Geometry: final body of the model. Coordinates: model frame, mm. A direction names the side the tool comes from. Round coordinates to 2 decimals unless told otherwise and drop trailing zeros. Loops run counter-clockwise (first coordinate to the right, second up) from the corner with the lowest first, then second, coordinate; pieces in that order, holes last. Notation, with made-up numbers: M 4,65 L 62,65 A28 cw 62,93 Z; hole C -1,49 d5. An arc over 180 degrees is marked long. Return JSON: item names as keys, results as strings.
from build123d import *

# Parameters (mm, degrees)
F4_W     = 64.961583
F4_H     = 61.849
F4_W_2   = 38.670417
F4_H_2   = 56.769
F5_DEPTH = 1.524
F1_R     = 3.7973
F1_R_2   = 2.07645
F1_R_3   = 2.286
F6_DEPTH = 4.064
F7_DEPTH = 25.4


with BuildPart() as f5:
    # F4 (on Top) → F5 (new body)
    with BuildSketch(Plane.XY):
        with Locations((-58.240771, 19.304)):
            Rectangle(F4_W, F4_H)
        with Locations((-58.240772, 19.304)):
            Rectangle(F4_W_2, F4_H_2, mode=Mode.SUBTRACT)
    extrude(amount=F5_DEPTH)

    # F1 (on Top) → F6 (join)
    with BuildSketch(Plane.XY):
        with Locations((-84.910771, -5.08)):
            Circle(F1_R)
        with Locations((-84.910771, -5.08)):
            Circle(F1_R_2, mode=Mode.SUBTRACT)
        with Locations((-83.640771, 43.688)):
            Circle(F1_R_3)
        with Locations((-32.840771, 0)):
            Circle(F1_R_3)
        with Locations((-32.840771, 28.448)):
            Circle(F1_R)
        with Locations((-32.840771, 28.448)):
            Circle(F1_R_2, mode=Mode.SUBTRACT)
    extrude(amount=F6_DEPTH)

    # F1 (on Top) → F7 (cut)
    with BuildSketch(Plane.XY):
        with Locations((-84.910771, -5.08)):
            Circle(F1_R_2)
        with Locations((-32.840771, 28.448)):
            Circle(F1_R_2)
    extrude(amount=F7_DEPTH, mode=Mode.SUBTRACT)


solid = f5.part
Q1. Section query D-D (z = 3.25). Output: boundary loops of the cut face in (x, y).
Determined:
{"outline": "C -84.91,-5.08 d7.59; C -83.64,43.69 d4.57; C -32.84,28.45 d7.59; C -32.84,0 d4.57; hole C -84.91,-5.08 d4.15; hole C -32.84,28.45 d4.15"}
Q2. Pin query (flat end, axial travel): pin 1 (10 mm diameter, centred on x = -32.5, y = 13.5, fed in from +Z); pin 2 (2 mm diameter, centred on y = 28.5, z = 3, fed in from -X); pin 3 (1.5 mm diameter, centred on y = 19.5, z = 3, fed in from +X). Return the tip coordinate at first contact, or that it passes through.
Determined:
{"pin 1": "stops at z = 1.52", "pin 2": "stops at x = -36.64", "pin 3": "passes through"}
Q3. Material intervals for L1, parallel to Y at x = -55.5, z = 1.15; L2, parallel to X at y = 8.5, z = 0.65; L3, parallel to Y at x = -83, z = 2.1, sorted ascending.
Determined:
{"L1": "y = -11.62 to -9.08, 47.69 to 50.23", "L2": "x = -90.72 to -77.58, -38.91 to -25.76", "L3": "y = -8.36 to -5.89, -4.27 to -1.8, 41.49 to 45.88"}
Q4. Pull-direction query (Y, two-part tool) for faces 1 (the flat face through (-38.906, 19, 1)), 2 (the flat face through (-59, -11.62, 1)), 3 (the flat face through (-31, 27, 4.064)); classes: pulls with the +Y half, pulls with the -Y half, needs draft (parallel to the pull), parting line crosses it, or undercut.
Determined:
{"face 1": "undercut", "face 2": "pulls with the -Y half", "face 3": "needs draft"}
Q5. Section query B-B (x = -50). Output: boundary loops of the cut face in (y, z), plus the area to 3 significant figures.
Determined:
{"outline": "M -11.62,0 L -9.08,0 L -9.08,1.52 L -11.62,1.52 Z; M 47.69,0 L 50.23,0 L 50.23,1.52 L 47.69,1.52 Z", "area": "7.74 mm^2"}
Q6. Reachability of faces 4 (the flat face through (-59, 47.688, 1)), 5 (the cylindrical face through (-81.3, -3.9, 2.8)), 6 (the flat face through (-83, -7, 4.064)) from +Z, -Z, +X, -X, +Y, -Y: full face, straight path, thin tool, end or side. Return the list, or none.
Determined:
{"face 4": "+Z, -Z", "face 5": "+Z", "face 6": "+Z, +X, -X, +Y, -Y"}
Q7. Section query C-C (y = 40). Output: boundary loops of the cut face in (x, z).
Determined:
{"outline": "M -90.72,0 L -77.58,0 L -77.58,1.52 L -90.72,1.52 Z; M -38.91,0 L -25.76,0 L -25.76,1.52 L -38.91,1.52 Z"}
Q8. Section query A-A (y = -5.08). Output: boundary loops of the cut face in (x, z), plus the area to 3 significant figures.
Determined:
{"outline": "M -90.72,0 L -86.99,0 L -86.99,4.06 L -88.71,4.06 L -88.71,1.52 L -90.72,1.52 Z; M -82.83,0 L -77.58,0 L -77.58,1.52 L -81.11,1.52 L -81.11,4.06 L -82.83,4.06 Z; M -38.91,0 L -25.76,0 L -25.76,1.52 L -38.91,1.52 Z", "area": "42.5 mm^2"}
